from build123d import *

# Parameters (mm, degrees)
BOSS_EXTRUDE1_DEPTH   = 25
BOSS_EXTRUDE1_2_DEPTH = 25
BOSS_EXTRUDE2_REACH   = 58.352
SKETCH2_W             = 10
SKETCH2_H             = 7.109401076
BOSS_EXTRUDE3_DEPTH   = 10
SKETCH4_R             = 2.5
CUT_EXTRUDE1_DEPTH    = 66.828745993


with BuildPart() as part:
    # Sketch1 → Boss-Extrude1 (new body)
    with BuildSketch(Plane.XY):
        Polygon((-6.156921938, -3.554700538), (0, -7.109401077), (6.156921938, -3.554700538), (6.156921938, 3.554700538), (0, 7.109401077), (-6.156921938, 3.554700538), align=None)
        Polygon((-4.156921938, 2.4), (-4.156921938, -2.4), (0, -4.8), (4.156921938, -2.4), (4.156921938, 2.4), (0, 4.8), align=None, mode=Mode.SUBTRACT)
    extrude(amount=BOSS_EXTRUDE1_DEPTH)


with BuildPart() as body_2:
    # Sketch1 → Boss-Extrude1 2 (new body)
    with BuildSketch(Plane.XY):
        Polygon((43.843078062, -3.554700538), (50, -7.109401077), (56.156921938, -3.554700538), (56.156921938, 3.554700538), (50, 7.109401077), (43.843078062, 3.554700538), align=None)
        Polygon((45.843078062, -2.4), (50, -4.8), (54.156921938, -2.4), (54.156921938, 2.4), (50, 4.8), (45.843078062, 2.4), align=None, mode=Mode.SUBTRACT)
    extrude(amount=BOSS_EXTRUDE1_2_DEPTH)

    # Boss-Extrude2: up to this face of the body (flat: up to its plane)
    boss_extrude2_end = Plane(body_2.part.faces().sort_by_distance((43.843078062, 0, 12.5))[0])
    # Sketch2 → Boss-Extrude2 (add, up to the picked face)
    with BuildSketch(Plane(origin=(6.156921938, 0, 0), x_dir=(0, 0, -1), z_dir=(1, 0, 0)), mode=Mode.PRIVATE) as boss_extrude2_sk1:
        with Locations((-20, 0)):
            Rectangle(SKETCH2_W, SKETCH2_H)
    boss_extrude2_tool1 = split(extrude(boss_extrude2_sk1.sketch, amount=BOSS_EXTRUDE2_REACH, mode=Mode.PRIVATE), bisect_by=boss_extrude2_end, keep=Keep.BOTH, mode=Mode.PRIVATE)

    add(part.part)  # Boss-Extrude2 merges part
    add(boss_extrude2_tool1.solids().sort_by(Axis((6.156922, 0, 20), (1, 0, 0)))[0])

    # Sketch3 → Boss-Extrude3 (add)
    with BuildSketch(Plane.XY.offset(25)):
        Polygon((50, 7.109401077), (50, 23.554700538), (0, 23.554700538), (0, 7.109401077), (6.156921938, 3.554700538), (43.843078062, 3.554700538), align=None)
    extrude(amount=-BOSS_EXTRUDE3_DEPTH)

    # Sketch4 → Cut-Extrude1 (cut, through all)
    with BuildSketch(Plane.XY.offset(25)):
        with Locations((25, 17.554700538)):
            Circle(SKETCH4_R)
        with Locations((35, 17.554700538)):
            Circle(SKETCH4_R)
        with Locations((45, 17.554700538)):
            Circle(SKETCH4_R)
        with Locations((15, 17.554700538)):
            Circle(SKETCH4_R)
        with Locations((5, 17.554700538)):
            Circle(SKETCH4_R)
    extrude(amount=-CUT_EXTRUDE1_DEPTH, mode=Mode.SUBTRACT)


solid = body_2.part
Geometry check sheet. Reference: the model listing, model coordinates, mm. A direction names the side the tool comes from. Give positions to 0.01 mm unless a question says otherwise; leave off trailing zeros. Order: outer loops, then holes, each group sorted by start corner. A loop starts at its lowest first (then second) coordinate and runs counter-clockwise, first axis right, second up.
1. Sectioned sample at D-D (y = 16.5). Record the boundary of the cut face in (x, z), then the cut area to 3 significant figures.
Completed:
outline: (0, 15) - (2.73, 15) - (2.73, 25) - (0, 25) - close; (7.27, 15) - (12.73, 15) - (12.73, 25) - (7.27, 25) - close; (17.27, 15) - (22.73, 15) - (22.73, 25) - (17.27, 25) - close; (27.27, 15) - (32.73, 15) - (32.73, 25) - (27.27, 25) - close; (37.27, 15) - (42.73, 15) - (42.73, 25) - (37.27, 25) - close; (47.27, 15) - (50, 15) - (50, 25) - (47.27, 25) - close
area: 273 mm2
2. Sectioned sample at B-B (y = 0). Record the boundary of the cut face in (x, z).
Completed:
outline: (-6.16, 0) - (-4.16, 0) - (-4.16, 25) - (-6.16, 25) - close; (4.16, 0) - (6.16, 0) - (6.16, 15) - (43.84, 15) - (43.84, 0) - (45.84, 0) - (45.84, 25) - (4.16, 25) - close; (54.16, 0) - (56.16, 0) - (56.16, 25) - (54.16, 25) - close
3. Draft check along X on faces 1 (the face through (50, 15, 20)), 2 (the face through (6.344, 19.663, 20.07)), 3 (the face through (-3.035, 5.357, 12.325)), 4 (the face through (23.157, 19.244, 20.07)). Enter one of: pulls with the +X half, pulls with the -X half, needs draft (parallel to the pull), parting line crosses it, or undercut.
Completed:
face 1: pulls with the +X half
face 2: undercut
face 3: pulls with the -X half
face 4: undercut
4. Access from +Z, -Z, +X, -X, +Y, -Y to the whole of each face (thin tool, end or side, straight path). Record for faces 5 (the face through (-1, -5, 0)), 6 (the face through (46.965, 5.357, 7.395)), 7 (the face through (25, -3.555, 20)), 8 (the face through (52.049, -3.617, 12.325)), 9 (the face through (-3.12, -5.31, 12.32)).
Completed:
face 5: -Z, +X, -X, +Y, -Y
face 6: -Z, +Y
face 7: +Z, -Z, -Y
face 8: +Z, -Z
face 9: +Z, -Z, -X, -Y
5. Sectioned sample at C-C (x = 25). Record the boundary of the cut face in (y, z), then the cut area to 3 significant figures.
Completed:
outline: (-3.55, 15) - (15.05, 15) - (15.05, 25) - (-3.55, 25) - close; (20.05, 15) - (23.55, 15) - (23.55, 25) - (20.05, 25) - close
area: 221 mm2
6. Depth check by flat-ended pin: pin 1 (1.5 mm diameter, centred on x = 12, y = -3.5, fed in from -Z); pin 2 (11 mm diameter, centred on y = 11.5, z = 22, fed in from +X); pin 3 (5 mm diameter, centred on x = 32.5, z = 20.5, fed in from -Y). Enter the tip coordinate at first touch or a pass-through.
Completed:
pin 1: stops at z = 15
pin 2: stops at x = 51.92
pin 3: stops at y = -3.55
7. Sectioned sample at A-A (z = 3.5). Record the boundary of the cut face in (x, y).
Completed:
outline: (-6.16, -3.55) - (0, -7.11) - (6.16, -3.55) - (6.16, 3.55) - (0, 7.11) - (-6.16, 3.55) - close; (43.84, -3.55) - (50, -7.11) - (56.16, -3.55) - (56.16, 3.55) - (50, 7.11) - (43.84, 3.55) - close; hole (-4.16, -2.4) - (0, -4.8) - (4.16, -2.4) - (4.16, 2.4) - (0, 4.8) - (-4.16, 2.4) - close; hole (45.84, -2.4) - (50, -4.8) - (54.16, -2.4) - (54.16, 2.4) - (50, 4.8) - (45.84, 2.4) - close
8. Scan lines: line 1 (X direction, y = 0, z = 7.25); line 2 (Y direction, x = 25, z = 18.5); line 3 (Z direction, x = 46.5, y = 20). Record each from-to range of solid material in increasing order.
Completed:
line 1: x = -6.16 to -4.16, 4.16 to 6.16, 43.84 to 45.84, 54.16 to 56.16
line 2: y = -3.55 to 15.05, 20.05 to 23.55
line 3: z = 15 to 25
